Verification items for the finished model (mm, model axes). Face numbers are marked on the shaded views. A direction names the side the tool comes from. Coordinates: 2 decimals unless noted, no trailing zeros. Write each loop counter-clockwise with the first axis right and the second up, starting at its lowest first coordinate (ties: lowest second). Pieces come first, ordered by that corner, then holes. Notation, with made-up numbers: M 84,10.25 L 96,10.25 A18 cw 96,27.25 Z; hole C 2,58 d11. An arc over 180 degrees is marked long. Answer in a Markdown table with one row per item.
from build123d import *

# Parameters (mm, degrees)
F0_R     = 6.096
F0_R_2   = 5.1435
F1_DEPTH = 9.525
F2_R     = 6.35
F2_R_2   = 5.1435
F3_DEPTH = 2.54
F4_R     = 6.35
F4_R_2   = 5.1435
F5_DEPTH = 2.54
F6_SIZE  = 0.25399


# Not quite as in the source:
# - a fillet or chamfer is up to 0.001 mm smaller than in the source, because OpenCascade refuses the exact size


with BuildPart() as f1:
    # F0 (on Top) → F1 (new body)
    with BuildSketch(Plane.XY):
        Circle(F0_R)
        Circle(F0_R_2, mode=Mode.SUBTRACT)
    extrude(amount=F1_DEPTH)

    # F2 (on face) → F3 (join)
    with BuildSketch(Plane.XY.offset(9.525)):
        Circle(F2_R)
        Circle(F2_R_2, mode=Mode.SUBTRACT)
    extrude(amount=-F3_DEPTH)

    # F4 (on face) → F5 (join)
    with BuildSketch(Plane(origin=(0, 0, 0), x_dir=(1, 0, 0), z_dir=(0, 0, -1))):
        Circle(F4_R)
        Circle(F4_R_2, mode=Mode.SUBTRACT)
    extrude(amount=-F5_DEPTH)

    # F6 (size 0.254 in the source; OpenCascade refuses exactly that, so slightly less here)
    f6_edges = [f1.edges().sort_by_distance(p)[0] for p in [
        (-6.35, 0, 6.985),
        (-6.35, 0, 9.525),
        (-6.35, 0, 2.54),
        (-6.35, 0, 0),
    ]]
    chamfer(f6_edges, length=F6_SIZE)


solid = f1.part
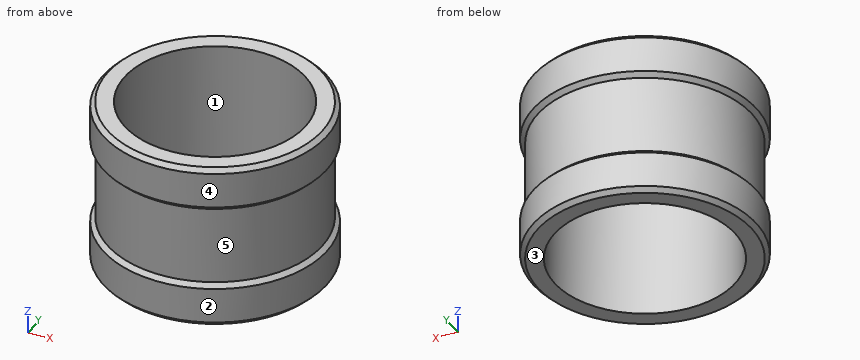
1) Sectioned sample at C-C (z = 7.75). Record the cut outline in (x, y), then the cut area to 3 significant figures.
Response values:
| item | result |
|---|---|
| outline | C 0,0 d12.7; hole C 0,0 d10.29 |
| area | 43.6 mm² |
2) Thickness scan on L1, parallel to Y at x = 0, z = 7.5; L2, parallel to Y at x = 0, z = 3.25; L3, parallel to X at y = 2, z = 1.75. Record the ranges inside material, lowest first. Write a range as [from, to].
Response values:
| item | result |
|---|---|
| L1 | y = [-6.35, -5.14], [5.14, 6.35] |
| L2 | y = [-6.1, -5.14], [5.14, 6.1] |
| L3 | x = [-6.03, -4.74], [4.74, 6.03] |
3) Depth check by flat-ended pin: pin 1 (1.5 mm diameter, centred on y = 1.5, z = 5, fed in from +X); pin 2 (2 mm diameter, centred on x = -2, y = -4.5, fed in from +Z) (3 decimals); pin 3 (5 mm diameter, centred on x = 3.5, z = 5, fed in from +Y); pin 4 (3.5 mm diameter, centred on x = -2, y = -1, fed in from -Z). Enter the tip coordinate at first touch or a pass-through.
Response values:
| item | result |
|---|---|
| pin 1 | stops at x = 6.05 |
| pin 2 | stops at z = 9.525 |
| pin 3 | stops at y = 6.01 |
| pin 4 | passes through |
4) Sectioned sample at D-D (z = 5.25). Record the cut outline in (x, y).
Response values:
| item | result |
|---|---|
| outline | C 0,0 d12.19; hole C 0,0 d10.29 |
5) Tool access check on the marked faces 4 and 5. Record the directions out of +Z, -Z, +X, -X, +Y, -Y that give a thin tool (end or side, any length) a straight path to the whole face; none if there is none.
Response values:
| item | result |
|---|---|
| face 4 | +Z, -Z |
| face 5 | none |
6) Release check for a two-part mould opening along X. For the marked faces 1, 2 and 3 record: +X half, -X half, draft (parallel to the pull), parting line (faces both ways), or undercut.
Response values:
| item | result |
|---|---|
| face 1 | undercut |
| face 2 | parting line |
| face 3 | draft |
